Build history of the part. All positions in model axes, mm. A direction names the side the tool comes from. Round coordinates to 2 decimals unless told otherwise and drop trailing zeros. Write each loop counter-clockwise with the first axis right and the second up, starting at its lowest first coordinate (ties: lowest second). Pieces come first, ordered by that corner, then holes. Notation, with made-up numbers: (83, 84) - (129, 84) arc R18 cw to (129, 97) - close; hole circle Ø8 at (-28, 55.25). An arc over 180 degrees is marked (long way). One line per question, with ' | ' between items.
from build123d import *

# Parameters (mm, degrees)
SKETCH_1_R          = 16.5
EXTRUDE_1_DEPTH     = 68
CHAMFER_1_SIZE      = 1
SKETCH_3_R          = 6
EXTRUDE_2_DEPTH     = 14
CUT_EXTRUDE_3_DEPTH = 6


with BuildPart() as part:
    # 草圖1 → 伸長1 (new body)
    with BuildSketch(Plane.XY):
        Circle(SKETCH_1_R)
    extrude(amount=EXTRUDE_1_DEPTH)

    # 導角1
    chamfer_1_edges = [part.edges().sort_by_distance(p)[0] for p in [
        (-16.5, 0, 68),
    ]]
    chamfer(chamfer_1_edges, length=CHAMFER_1_SIZE)

    # 草圖3 → 伸長2 (add, symmetric)
    with BuildSketch(Plane(origin=(0, 0, 0), x_dir=(0, 0, -1), z_dir=(1, 0, 0))):
        with BuildLine():
            Line((0, 14), (19, 14))
            ThreePointArc((19, 14), (33, 0), (19, -14))
            Line((19, -14), (0, -14))
            Line((0, -14), (0, 14))
        make_face()
        with Locations((19, 0)):
            Circle(SKETCH_3_R, mode=Mode.SUBTRACT)
    extrude(amount=EXTRUDE_2_DEPTH, both=True)

    # 草圖4 → 伸長3 (cut, symmetric)
    with BuildSketch(Plane(origin=(0, 0, 0), x_dir=(0, 0, -1), z_dir=(1, 0, 0))):
        with BuildLine():
            Line((3, 14), (3, -14))
            Line((3, -14), (19, -14))
            ThreePointArc((19, -14), (33, 0), (19, 14))
            Line((19, 14), (3, 14))
        make_face()
    extrude(amount=CUT_EXTRUDE_3_DEPTH, both=True, mode=Mode.SUBTRACT)


solid = part.part
Q1. Which spindle directions (+Z, -Z, +X, -X, +Y, -Y) get a long thin tool onto all of the face, cutting with end or side? Do faces 1 (the flat face through (14, 3, -13)), 2 (the flat face through (-14, 3, -13)), 3 (the flat face through (-6, 0, -11)), 4 (the flat face through (6.4, -14, -9.6)), 5 (the flat face through (13, -13, 0)). Say none if no direction does.
Found:
face 1: -Z, +X, +Y, -Y | face 2: -Z, -X, +Y, -Y | face 3: -Z, +Y, -Y | face 4: -Z, +X, -X, -Y | face 5: +Z, +X, -Y
Q2. Saw through at B-B, the plane z = -5.5. List the corners of the cut face in (x, y).
Found:
outline: (-14, -14) - (-6, -14) - (-6, 14) - (-14, 14) - close; (6, -14) - (14, -14) - (14, 14) - (6, 14) - close
Q3. Drill centre lines: L1, parallel to X at y = -6, z = -4; L2, parallel to Y at x = -10, z = -7. Where is each one in solid material? Low to high. Write a range as from..to.
Found:
L1: -14..-6, 6..14 | L2: -14..14
Q4. Drop flat-ended pins along their axis: pin 1 (5.5 mm diameter, centred on x = -6.5, z = -10, fed in from -Y); pin 2 (8.5 mm diameter, centred on y = 3, z = -17, fed in from +X); pin 3 (14 mm diameter, centred on y = 6.5, z = -21, fed in from -X); pin 4 (11 mm diameter, centred on y = 0, z = -19, fed in from +X). Give the stop position or say it passes through.
Found:
pin 1: y = -14 | pin 2: x = 14 | pin 3: x = -14 | pin 4: through
Q5. Pull direction Y, two halves, no side cores. Call faces 6 (the cylindrical face through (10, 0, -33)), 7 (the cylindrical face through (9.94, -2.3, -24.54)), 8 (the flat face through (13, 12, 0)), 9 (the cylindrical face through (-10.06, -2.3, -24.54)): +Y half, -Y half, draft (parallel to the pull), parting line (faces both ways), or undercut.
Found:
face 6: parting line | face 7: undercut | face 8: draft | face 9: undercut
Q6. Saw through at A-A, the plane y = 0. List the corners of the cut face in (x, z).
Found:
outline: (-16.5, 0) - (-14, 0) - (-14, -13) - (-6, -13) - (-6, -3) - (6, -3) - (6, -13) - (14, -13) - (14, 0) - (16.5, 0) - (16.5, 67) - (15.5, 68) - (-15.5, 68) - (-16.5, 67) - close; (-14, -33) - (-6, -33) - (-6, -25) - (-14, -25) - close; (6, -33) - (14, -33) - (14, -25) - (6, -25) - close
Q7. Saw through at D-D, the plane z = 21. List the corners of the cut face in (x, y), then the cut area to 3 significant figures.
Found:
outline: circle Ø33 at (0, 0) | area: 855 mm^2
Q8. Saw through at C-C, the plane x = 0. List the corners of the cut face in (y, z), then the cut area to 3 significant figures.
Found:
outline: (-16.5, 0) - (-14, 0) - (-14, -3) - (14, -3) - (14, 0) - (16.5, 0) - (16.5, 67) - (15.5, 68) - (-15.5, 68) - (-16.5, 67) - close | area: 2,330 mm^2
